from build123d import *

# Parameters (mm, degrees)
F0_W     = 88.9
F0_H     = 38.1
F1_DEPTH = 311.15
F2_R     = 9.525
F3_DEPTH = 12.7


with BuildPart() as f1:
    # F0 (on Front) → F1 (new body, symmetric)
    with BuildSketch(Plane.XZ):
        Rectangle(F0_W, F0_H)
    extrude(amount=F1_DEPTH, both=True)

    # F2 (on face) → F3 (cut)
    with BuildSketch(Plane(origin=(0, 0, -19.05), x_dir=(1, 0, 0), z_dir=(0, 0, -1))):
        with Locations((0, 266.7)):
            Circle(F2_R)
        with Locations((0, -266.7)):
            Circle(F2_R)
    extrude(amount=-F3_DEPTH, mode=Mode.SUBTRACT)


solid = f1.part
Design review of the part built by this model. Coordinates are the model's own, in mm. A direction names the side the tool comes from. Give positions to 0.01 mm unless a question says otherwise; leave off trailing zeros. Order: outer loops, then holes, each group sorted by start corner. A loop starts at its lowest first (then second) coordinate and runs counter-clockwise, first axis right, second up.
1. Add section B-B, the plane y = -266.7. State the section outline as (x, z) points (3 decimals).
Solution:
outline: (-44.45, -19.05) - (-9.525, -19.05) - (-9.525, -6.35) - (9.525, -6.35) - (9.525, -19.05) - (44.45, -19.05) - (44.45, 19.05) - (-44.45, 19.05) - close
2. Add section A-A, the plane x = 0. State the section outline as (y, z) points (3 decimals), then the cut area to 3 significant figures.
Solution:
outline: (-311.15, -19.05) - (-276.225, -19.05) - (-276.225, -6.35) - (-257.175, -6.35) - (-257.175, -19.05) - (257.175, -19.05) - (257.175, -6.35) - (276.225, -6.35) - (276.225, -19.05) - (311.15, -19.05) - (311.15, 19.05) - (-311.15, 19.05) - close
area: 23,200 mm2
3. To check wall thickness, follow L1, parallel to Y at x = 0, z = -15 (3 decimals); L2, parallel to X at y = -266.7, z = -15.75 (3 decimals). State the ranges of each line that lie inside material, in increasing order.
Solution:
L1: y = -311.15 to -276.225, -257.175 to 257.175, 276.225 to 311.15
L2: x = -44.45 to -9.525, 9.525 to 44.45
4. Tool access review of faces 1 (the flat face through (-1, 311.15, 0)), 2 (the cylindrical face through (-2.06, 276, -12.79)): name each direction out of +Z, -Z, +X, -X, +Y, -Y from which nothing blocks a thin tool from reaching the whole face with its end or side.
Solution:
face 1: +Z, -Z, +X, -X, +Y
face 2: -Z
5. Mouldability with a two-part tool opening along Y and no side actions: class faces 3 (the flat face through (0, 267, -6.35)), 4 (the flat face through (-1, -311.15, 0)), 5 (the flat face through (-1, -4, -19.05)) as +Y half, -Y half, draft (parallel to the pull), parting line (faces both ways), or undercut.
Solution:
face 3: undercut
face 4: -Y half
face 5: draft
6. For pin 1 Ø5.5 at (x, y) = (-0.5, -265) entering from -Z, flat-tipped, find the tip position at first contact; note if it passes through.
Solution:
pin 1: stops at z = -6.35
